from build123d import *

# Parameters (mm, degrees)
F0_R     = 38.1
F1_DEPTH = 6.35
F2_R     = 38.1
F2_R_2   = 31.75
F3_DEPTH = 152.4
F4_R     = 3.17499


# Not quite as in the source:
# - a fillet or chamfer is up to 0.001 mm smaller than in the source, because OpenCascade refuses the exact size


with BuildPart() as f1:
    # F0 (on Top) → F1 (new body)
    with BuildSketch(Plane.XY):
        with Locations((-62.3559355736, 26.823958382)):
            Circle(F0_R)
    extrude(amount=F1_DEPTH)

    # F2 (on face) → F3 (join)
    with BuildSketch(Plane.XY.offset(6.35)):
        with Locations((-62.3559355736, 26.823958382)):
            Circle(F2_R)
        with Locations((-62.3559355736, 26.823958382)):
            Circle(F2_R_2, mode=Mode.SUBTRACT)
    extrude(amount=F3_DEPTH)

    # F4 (radius 3.175 in the source; OpenCascade refuses exactly that, so slightly less here)
    f4_edges = [f1.edges().sort_by_distance(p)[0] for p in [
        (-94.105936, 26.823958, 158.75),
        (-100.455936, 26.823958, 158.75),
    ]]
    fillet(f4_edges, radius=F4_R)


solid = f1.part
The model under review builds one solid part; all positions refer to its coordinate system, in mm. Round coordinates to 2 decimals unless told otherwise and drop trailing zeros. Loops run counter-clockwise (first coordinate to the right, second up) from the corner with the lowest first, then second, coordinate; pieces in that order, holes last. Notation, with made-up numbers: (-4, -23) -> (6, -23) arc R15 cw to (6, -6) -> close; hole circle Ø3 at (27.5, -25). An arc over 180 degrees is marked (long way). Write item = value, one per line. Start each with the question number.
Item 1: Mouldability with a two-part tool opening along Y and no side actions: class faces 1 (the cylindrical face through (-92.59, 3.64, 76.7)), 2 (the flat face through (-63, 27, 6.35)), 3 (the cylindrical face through (-69.24, -4.17, 79.92)), 4 (the flat face through (-63, 27, 0)) as released by +Y, released by -Y, zero draft, split by the parting line, or undercut.
Item 2: To check wall thickness, follow L1, parallel to X at y = 25.5, z = 143.5; L2, parallel to Z at x = -71.5, y = 6.5; L3, parallel to X at y = 14, z = 118. State the ranges of each line that lie inside material, in increasing order.
Item 3: Insertion check: pin 1 (3 mm diameter, centred on y = 22.5, z = 30, fed in from +X); pin 2 (1 mm diameter, centred on x = -85.5, y = 8.5, fed in from +Z); pin 3 (4 mm diameter, centred on x = -41.5, z = 43, fed in from +Y). Each pin has a flat end and moves straight along its axis. Give the tip position at first contact, or say it passes through.
Item 4: Take a section at A-A on z = 45. Give the boundary of the cut face in (x, y), plus the area to 3 significant figures.
Result:
q1.face_1 = split by the parting line
q1.face_2 = undercut
q1.face_3 = undercut
q1.face_4 = zero draft
q2.L1 = -100.43 to -94.08, -30.63 to -24.28
q2.L2 = 0 to 6.35
q2.L3 = -98.23 to -91.4, -33.31 to -26.48
q3.pin_1 = -24.36
q3.pin_2 = 6.35
q3.pin_3 = 59.93
q4.outline = circle Ø76.2 at (-62.36, 26.82); hole circle Ø63.5 at (-62.36, 26.82)
q4.area = 1,390 mm²
